Could you check a few things on this drawing? It's one solid part, dimensions in mm from its lowest x, y, z. A direction names the side the tool comes from. Round coordinates to 2 decimals unless told otherwise and drop trailing zeros. Loops run counter-clockwise (first coordinate to the right, second up) from the corner with the lowest first, then second, coordinate; pieces in that order, holes last. Notation, with made-up numbers: (-6, 25) -> (42, 25) arc R21 ccw to (42, 29) -> close; hole circle Ø4 at (52, -30). An arc over 180 degrees is marked (long way). Write each question's results on one line, items separated by ' | '.
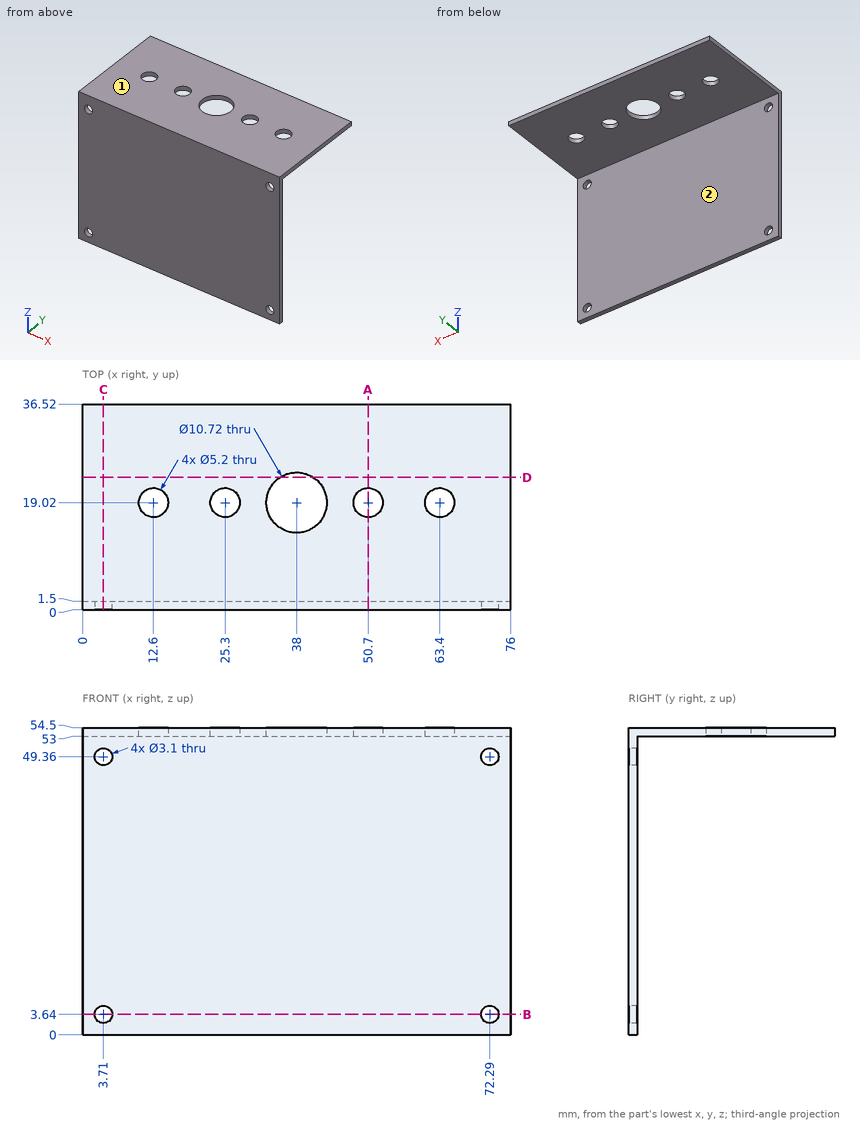
1) I need wall thicknesses on line 1 (X direction, y = 0.45, z = 49.36); line 2 (Y direction, x = 19, z = 51.5); line 3 (X direction, y = 1, z = 3). Which ranges of each line are inside material? Lowest first, please.
Model answer:
line 1: x = 0 to 2.16, 5.26 to 70.74, 73.84 to 76 | line 2: y = 0 to 1.5 | line 3: x = 0 to 2.3, 5.12 to 70.88, 73.7 to 76
2) I'm going to push flat-ended pins straight in: pin 1 (1.5 mm diameter, centred on x = 66, z = 29, fed in from -Y); pin 2 (12 mm diameter, centred on x = 49.5, y = 26, fed in from -Z); pin 3 (10 mm diameter, centred on x = 63, z = 44, fed in from +Y). Where does each tip first touch, or does it pass through?
Model answer:
pin 1: stops at y = 0 | pin 2: stops at z = 53 | pin 3: stops at y = 1.5
3) I want a section at C-C, the plane x = 3.71. Write out the boundary of the cut face in (y, z).
Model answer:
outline: (0, 0) -> (1.5, 0) -> (1.5, 2.09) -> (0, 2.09) -> close; (0, 5.19) -> (1.5, 5.19) -> (1.5, 47.81) -> (0, 47.81) -> close; (0, 50.91) -> (1.5, 50.91) -> (1.5, 53) -> (36.52, 53) -> (36.52, 54.5) -> (0, 54.5) -> close
4) For the marked faces 1 and 2, which set-ups out of +Z, -Z, +X, -X, +Y, -Y let a thin tool reach every point of the face, with its end or its side?
Model answer:
face 1: +Z, +X, -X, +Y, -Y | face 2: -Z, +X, -X, +Y
5) I want a section at D-D, the plane y = 23.5. Write out the boundary of the cut face in (x, z), plus the area to 3 significant figures.
Model answer:
outline: (0, 53) -> (35.06, 53) -> (35.06, 54.5) -> (0, 54.5) -> close; (40.94, 53) -> (76, 53) -> (76, 54.5) -> (40.94, 54.5) -> close | area: 105 mm2
6) I want a section at A-A, the plane x = 50.7. Write out the boundary of the cut face in (y, z), plus the area to 3 significant figures.
Model answer:
outline: (0, 0) -> (1.5, 0) -> (1.5, 53) -> (16.42, 53) -> (16.42, 54.5) -> (0, 54.5) -> close; (21.62, 53) -> (36.52, 53) -> (36.52, 54.5) -> (21.62, 54.5) -> close | area: 126 mm2
7) I want a section at B-B, the plane z = 3.64. Write out the boundary of the cut face in (x, y), plus the area to 3 significant figures.
Model answer:
outline: (0, 0) -> (2.16, 0) -> (2.16, 1.5) -> (0, 1.5) -> close; (5.26, 0) -> (70.74, 0) -> (70.74, 1.5) -> (5.26, 1.5) -> close; (73.84, 0) -> (76, 0) -> (76, 1.5) -> (73.84, 1.5) -> close | area: 105 mm2
